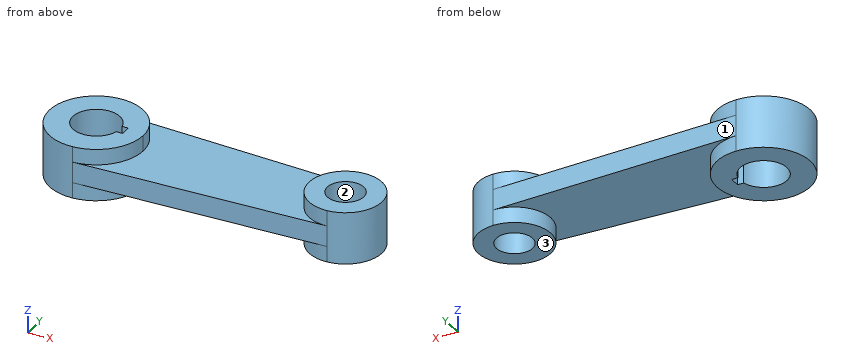
from build123d import *

# Parameters (mm, degrees)
F0_R          = 21.9
F1_DEPTH      = 12.5
F1_DEPTH_BACK = 12.5
F2_R          = 21.9
F3_DEPTH      = 18.75


with BuildPart() as f1:
    # F0 (on Top) → F1 (new body, two sides)
    with BuildSketch(Plane.XY) as f1_sk:
        with BuildLine():
            Line((151.822917, 43.712006), (-147.65625, 56.201151))
            ThreePointArc((-147.65625, 56.201151), (-206.25, 0), (-147.65625, -56.201151))
            Line((-147.65625, -56.201151), (151.822917, -43.712006))
            ThreePointArc((151.822917, -43.712006), (193.75, 0), (151.822917, 43.712006))
        make_face()
        with BuildLine():
            ThreePointArc((-122.564029, -6.3), (-178.15, 0), (-122.564029, 6.3))
            Line((-122.564029, 6.3), (-115, 6.3))
            Line((-115, 6.3), (-115, -6.3))
            Line((-115, -6.3), (-122.564029, -6.3))
        make_face(mode=Mode.SUBTRACT)
        with Locations((150, 0)):
            Circle(F0_R, mode=Mode.SUBTRACT)
    extrude(amount=F1_DEPTH)
    extrude(f1_sk.sketch, amount=-F1_DEPTH_BACK)

    # F2 (on face) → F3 (join)
    with BuildSketch(Plane.XY.offset(12.5)):
        with BuildLine():
            ThreePointArc((-147.65625, -56.201151), (-109.405059, -38.937299), (-93.75, 0))
            ThreePointArc((-93.75, 0), (-109.405059, 38.937299), (-147.65625, 56.201151))
            ThreePointArc((-147.65625, 56.201151), (-206.25, 0), (-147.65625, -56.201151))
        make_face()
        with BuildLine():
            ThreePointArc((-122.564029, -6.3), (-178.15, 0), (-122.564029, 6.3))
            Line((-122.564029, 6.3), (-115, 6.3))
            Line((-115, 6.3), (-115, -6.3))
            Line((-115, -6.3), (-122.564029, -6.3))
        make_face(mode=Mode.SUBTRACT)
        with BuildLine():
            ThreePointArc((193.75, 0), (181.573843, 30.284566), (151.822917, 43.712006))
            ThreePointArc((151.822917, 43.712006), (106.25, 0), (151.822917, -43.712006))
            ThreePointArc((151.822917, -43.712006), (181.573843, -30.284566), (193.75, 0))
        make_face()
        with Locations((150, 0)):
            Circle(F2_R, mode=Mode.SUBTRACT)
    extrude(amount=F3_DEPTH)

    # F4: F1 across plane


with BuildPart() as f1_1:
    add(f1.part)
    add(f1.part.mirror(Plane.XY))


solid = f1_1.part
For this review, take the finished solid that the model builds, in its own axes (mm). Face numbers are marked on the shaded views. Round coordinates to 2 decimals unless told otherwise and drop trailing zeros. Write each loop counter-clockwise with the first axis right and the second up, starting at its lowest first coordinate (ties: lowest second). Pieces come first, ordered by that corner, then holes. Notation, with made-up numbers: (-25.5, 15.25) - (2.5, 15.25) arc R30 cw to (2.5, 38.25) - close; hole circle Ø5 at (39.25, 85). An arc over 180 degrees is marked (long way). Use a Markdown table: item, result.
Q1. The part is to be moulded in two halves that separate along X. For the marked faces 1, 2 and 3, say which applies: pulls with the +X half, pulls with the -X half, needs draft (parallel to the pull), parting line crosses it, or undercut.
Derived:
| item | result |
|---|---|
| face 1 | pulls with the +X half |
| face 2 | undercut |
| face 3 | needs draft |
Q2. Wall thickness on line 1 along Y through (x, z) = (-150, 0); line 2 along Y through (x, z) = (150, -12.5); line 3 along X through (y, z) = (2, 19.5): over which ranges is each line inside the solid? List them lowest first.
Derived:
| item | result |
|---|---|
| line 1 | y = -56.25 to -28.15, 28.15 to 56.25 |
| line 2 | y = -43.75 to -21.9, 21.9 to 43.75 |
| line 3 | x = -206.21 to -178.08, -115 to -93.79, 106.3 to 128.19, 171.81 to 193.7 |
Q3. We need section B-B (y = 15). Give the boundary of the cut face in (x, z).
Derived:
| item | result |
|---|---|
| outline | (-204.21, -31.25) - (-173.82, -31.25) - (-173.82, 31.25) - (-204.21, 31.25) - close; (-126.18, -31.25) - (-95.79, -31.25) - (-95.79, -12.5) - (108.9, -12.5) - (108.9, -31.25) - (134.04, -31.25) - (134.04, 31.25) - (108.9, 31.25) - (108.9, 12.5) - (-95.79, 12.5) - (-95.79, 31.25) - (-126.18, 31.25) - close; (165.96, -31.25) - (191.1, -31.25) - (191.1, 31.25) - (165.96, 31.25) - close |
Q4. Clearance check with flat-ended pins moving along their axes: pin 1 (12 mm diameter, centred on y = 39, z = 0.5, fed in from +X); pin 2 (8 mm diameter, centred on x = 62, y = 32, fed in from +Z); pin 3 (5 mm diameter, centred on x = 8, z = 5.5, fed in from -Y); pin 4 (10 mm diameter, centred on x = 140.5, y = -13.5, fed in from +Z). State where each tip first meets the part, or that it passes through.
Derived:
| item | result |
|---|---|
| pin 1 | stops at x = 178.72 |
| pin 2 | stops at z = 12.5 |
| pin 3 | stops at y = -49.81 |
| pin 4 | passes through |
Q5. We need section A-A (z = -23). Give the boundary of the cut face in (x, y), plus the area to 3 significant figures.
Derived:
| item | result |
|---|---|
| outline | (-147.66, -56.2) arc R56.25 ccw to (-93.75, 0) arc R56.25 ccw to (-147.66, 56.2) arc R56.25 ccw (long way) to start; circle Ø87.5 at (150, 0); hole (-122.56, -6.3) - (-115, -6.3) - (-115, 6.3) - (-122.56, 6.3) arc R28.15 ccw (long way) to start; hole circle Ø43.8 at (150, 0) |
| area | 11,900 mm2 |
Q6. We need section D-D (x = -138.5). Give the boundary of the cut face in (y, z), plus the area to 3 significant figures.
Derived:
| item | result |
|---|---|
| outline | (-55.82, -12.5) - (-55.06, -12.5) - (-55.06, -31.25) - (-25.69, -31.25) - (-25.69, 31.25) - (-55.06, 31.25) - (-55.06, 12.5) - (-55.82, 12.5) - close; (25.69, -31.25) - (55.06, -31.25) - (55.06, -12.5) - (55.82, -12.5) - (55.82, 12.5) - (55.06, 12.5) - (55.06, 31.25) - (25.69, 31.25) - close |
| area | 3,710 mm2 |
Q7. We need section C-C (z = -6.5). Give the boundary of the cut face in (x, y), plus the area to 3 significant figures.
Derived:
| item | result |
|---|---|
| outline | (-147.66, -56.2) - (151.82, -43.71) arc R43.75 ccw to (151.82, 43.71) - (-147.66, 56.2) arc R56.25 ccw (long way) to start; hole (-122.56, -6.3) - (-115, -6.3) - (-115, 6.3) - (-122.56, 6.3) arc R28.15 ccw (long way) to start; hole circle Ø43.8 at (150, 0) |
| area | 33,900 mm2 |
